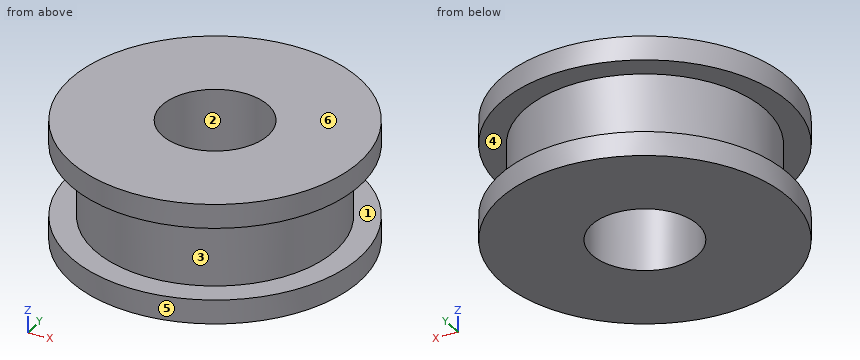
```python
from build123d import *

# Parameters (mm, degrees)
IZIM1_R                     = 25
Y_KSEKLIK_EKSTR_ZYON1_DEPTH = 15
IZIM3_R                     = 30
Y_KSEKLIK_EKSTR_ZYON2_DEPTH = 5
Y_KSEKLIK_EKSTR_ZYON3_START = 5
IZIM4_R                     = 30
Y_KSEKLIK_EKSTR_ZYON3_DEPTH = 5
IZIM5_R                     = 11
KES_EKSTR_ZYON1_DEPTH       = 50.244289009


with BuildPart() as part:
    # Çizim1 → Yükseklik-Ekstrüzyon1 (new body)
    with BuildSketch(Plane.XY):
        Circle(IZIM1_R)
    extrude(amount=Y_KSEKLIK_EKSTR_ZYON1_DEPTH)

    # Çizim3 → Yükseklik-Ekstrüzyon2 (add)
    with BuildSketch(Plane(origin=(0, 0, 0), x_dir=(-1, 0, 0), z_dir=(0, 0, -1))):
        Circle(IZIM3_R)
    extrude(amount=Y_KSEKLIK_EKSTR_ZYON2_DEPTH)

    # Çizim4 → Yükseklik-Ekstrüzyon3 (add)
    with BuildSketch(Plane.XY.offset(15).offset(Y_KSEKLIK_EKSTR_ZYON3_START)):
        with Locations(Location((0, 0, 0), (0, 0, 180))):
            Circle(IZIM4_R)
    extrude(amount=-Y_KSEKLIK_EKSTR_ZYON3_DEPTH)

    # Çizim5 → Kes-Ekstrüzyon1 (cut, through all)
    with BuildSketch(Plane.XY.offset(20)):
        Circle(IZIM5_R)
    extrude(amount=-KES_EKSTR_ZYON1_DEPTH, mode=Mode.SUBTRACT)


solid = part.part
```
Input: part model. Units: mm. Frame: model coordinates. Face numbers are marked on the shaded views. A direction names the side the tool comes from. Give positions to 0.01 mm unless a question says otherwise; leave off trailing zeros. Order: outer loops, then holes, each group sorted by start corner. A loop starts at its lowest first (then second) coordinate and runs counter-clockwise, first axis right, second up. Notation, with made-up numbers: M 83,58.25 L 95,58.25 A26 cw 95,84.25 Z; hole C 89,-30.5 d1. An arc over 180 degrees is marked long. Return JSON: item names as keys, results as strings.
Item 1: Cut plane C-C (z = 3.5). Return loops of the section in (x, y).
Solutions:
{"outline": "C 0,0 d50; hole C 0,0 d22"}
Item 2: Cut plane D-D (x = -17). Return loops of the section in (y, z), then the cut area to 3 significant figures.
Solutions:
{"outline": "M -24.72,-5 L 24.72,-5 L 24.72,0 L 18.33,0 L 18.33,15 L 24.72,15 L 24.72,20 L -24.72,20 L -24.72,15 L -18.33,15 L -18.33,0 L -24.72,0 Z", "area": "1,040 mm^2"}
Item 3: Access query for the marked faces 1 and 2. Directions: +Z, -Z, +X, -X, +Y, -Y. A direction counts if a zero-diameter tool reaches every point of the face in a straight line with its end or side. Return the directions, or none.
Solutions:
{"face 1": "none", "face 2": "+Z, -Z"}
Item 4: First-contact query: P1, Ø3, axis at y = 22, z = 8.5, coming from the +X side; P2, Ø8, axis at x = 15, z = 0, coming from the +Y side; P3, Ø4, axis at y = -13, z = -2.5, coming from the +X side; P4, Ø17.5, axis at x = 0, y = 0, coming from the +Z side. Flat tips, straight axial feed; report the tip coordinate or a pass-through.
Solutions:
{"P1": "x = 14.31", "P2": "y = 27.91", "P3": "x = 27.91", "P4": "through"}
Item 5: Ray query, probe 1 along Y at (x, z) = (0, 3.25); probe 2 along Z at (x, y) = (17, -24); probe 3 along X at (y, z) = (3, 9.5). Return the intervals inside material, ascending.
Solutions:
{"probe 1": "-25 to -11, 11 to 25", "probe 2": "-5 to 0, 15 to 20", "probe 3": "-24.82 to -10.58, 10.58 to 24.82"}
Item 6: Pull-direction query (Z, two-part tool) for the marked faces 3, 4, 5 and 6; classes: +Z half, -Z half, draft (parallel to the pull), parting line (faces both ways), or undercut.
Solutions:
{"face 3": "undercut", "face 4": "undercut", "face 5": "draft", "face 6": "+Z half"}
Item 7: Cut plane A-A (x = 0). Return loops of the section in (y, z), then the cut area to 3 significant figures.
Solutions:
{"outline": "M -30,-5 L -11,-5 L -11,20 L -30,20 L -30,15 L -25,15 L -25,0 L -30,0 Z; M 11,-5 L 30,-5 L 30,0 L 25,0 L 25,15 L 30,15 L 30,20 L 11,20 Z", "area": "800 mm^2"}
